```python
from build123d import *

# Parameters (mm, degrees)
F0_W     = 34.3586169891
F0_H     = 15
F1_DEPTH = 11.5
F2_DEPTH = 2.5
F3_DEPTH = 15
F5_DEPTH = 70
F6_R     = 1.75
F7_DEPTH = 50.001


with BuildPart() as f1:
    # F0 (on Top) → F1 (new body)
    with BuildSketch(Plane.XY):
        Rectangle(F0_W, F0_H)
    extrude(amount=F1_DEPTH)

    # F0 (on Top) → F2 (join)
    with BuildSketch(Plane.XY):
        Polygon((-43.5629601348, 31.9480635281), (-60, 31.9480635281), (-60, -31.9480635281), (-43.5629601348, -31.9480635281), (-17.1793084945, -13.474031764), (-17.1793084945, -10), (17.1793084945, -10), (17.1793084945, -13.474031764), (43.5629601348, -31.9480635281), (60, -31.9480635281), (60, 31.9480635281), (43.5629601348, 31.9480635281), (17.1793084945, 13.474031764), (17.1793084945, 10), (-17.1793084945, 10), (-17.1793084945, 13.474031764), align=None)
        Rectangle(F0_W, F0_H, mode=Mode.SUBTRACT)
    extrude(amount=F2_DEPTH)

    # F0 (on Top) → F3 (join)
    with BuildSketch(Plane.XY):
        Polygon((-43.5629601348, -31.9480635281), (-60, -31.9480635281), (-60, -35), (-43.5629601348, -35), (-15, -15), (15, -15), (43.5629601348, -35), (60, -35), (60, -31.9480635281), (43.5629601348, -31.9480635281), (17.1793084945, -13.474031764), (17.1793084945, -10), (-17.1793084945, -10), (-17.1793084945, -13.474031764), align=None)
        Polygon((15, 15), (-15, 15), (-43.5629601348, 35), (-60, 35), (-60, 31.9480635281), (-43.5629601348, 31.9480635281), (-17.1793084945, 13.474031764), (-17.1793084945, 10), (17.1793084945, 10), (17.1793084945, 13.474031764), (43.5629601348, 31.9480635281), (60, 31.9480635281), (60, 35), (43.5629601348, 35), align=None)
    extrude(amount=F3_DEPTH)

    # F4 (on face) → F5 (cut, through all)
    with BuildSketch(Plane.XZ.offset(35)):
        Polygon((-60, 15), (-60, 5), (-43.5629601348, 8.8385741302), (-43.5629601348, 15), align=None)
        Polygon((-43.5629601348, 15), (-43.5629601348, 8.8385741302), (-17.1793084945, 15), align=None)
        Polygon((17.1793084945, 15), (60, 5), (60, 15), align=None)
    extrude(amount=-F5_DEPTH, mode=Mode.SUBTRACT)

    # F6 (on face) → F7 (cut, through all)
    with BuildSketch(Plane.XZ.offset(15)):
        with Locations((-9.6793084945, 8.5)):
            Circle(F6_R)
        with Locations((9.6793084945, 8.5)):
            Circle(F6_R)
    extrude(amount=-F7_DEPTH, mode=Mode.SUBTRACT)


solid = f1.part
```
The listing builds one solid part. Answer for the finished solid, in the listing's coordinates (mm). A direction names the side the tool comes from. Give positions to 0.01 mm unless a question says otherwise; leave off trailing zeros. Order: outer loops, then holes, each group sorted by start corner. A loop starts at its lowest first (then second) coordinate and runs counter-clockwise, first axis right, second up. Notation, with made-up numbers: (4, 4) - (63, 4) arc R35 cw to (63, 40) - close; hole circle Ø7 at (-37, -37.5). An arc over 180 degrees is marked (long way). Answer in a Markdown table with one row per item. Add a question column.
Q1. Which of the six approach directions +Z, -Z, +X, -X, +Y, -Y give full straight-line access (tool end or side, diameter ignored) to faces 4 (the flat face through (0, -7.5, 7)), 5 (the flat face through (50, -31.948, 5)), 6 (the flat face through (-17.179, -12, 9))?
Q2. For a pull along Y with two mould halves and no side action, classify faces 1 (the flat face through (-52, -35, 3)), 2 (the flat face through (60, 0, 1)), 3 (the flat face through (-30.186, -22.582, 7.274)) as released by +Y, released by -Y, zero draft, split by the parting line, or undercut.
Q3. The part is cut by section D-D (x = -10). Determine the outline of the cut face in (y, z), then the cut area to 3 significant figures.
Q4. Find the intervals of material crossed by line 1 along Y through (x, z) = (-12, 7.25); line 2 along Y through (x, z) = (6.5, 11.75); line 3 along Z through (x, y) = (32, 1), in increasing order. Write a range as [from, to].
Q5. The part is cut by section A-A (y = 2). Determine the outline of the cut face in (x, z).
Q6. Given P1, Ø5, axis at y = 27.5, z = 7, coming from the -X side; P2, Ø12, axis at x = 45.5, y = 17.5, coming from the +Z side; P3, Ø2, axis at x = -9.68, z = 8.5, coming from the -Y side; P4, Ø1.5, axis at y = 22, z = 8, coming from the -X side, each flat-ended and moving along its own axis, determine where each tip first touches the part or whether it passes through.
Q7. The part is cut by section B-B (z = 12.75). Determine the outline of the cut face in (x, y).
Q8. The part is cut by section C-C (y = -21.5). Determine the outline of the cut face in (x, z), then the cut area to 3 significant figures.
Determined:
| question | item | result |
|---|---|---|
| 1 | face 4 | +Z, +X, -X |
| 1 | face 5 | +Z, +X |
| 1 | face 6 | +Z, -X |
| 2 | face 1 | released by -Y |
| 2 | face 2 | zero draft |
| 2 | face 3 | undercut |
| 3 | outline | (-15, 0) - (15, 0) - (15, 6.78) - (10, 6.78) - (10, 2.5) - (7.5, 2.5) - (7.5, 6.78) - (-7.5, 6.78) - (-7.5, 2.5) - (-10, 2.5) - (-10, 6.78) - (-15, 6.78) - close; (-15, 10.22) - (-10, 10.22) - (-10, 15) - (-15, 15) - close; (-7.5, 10.22) - (7.5, 10.22) - (7.5, 11.5) - (-7.5, 11.5) - close; (10, 10.22) - (15, 10.22) - (15, 15) - (10, 15) - close |
| 3 | area | 249 mm² |
| 4 | line 1 | y = [-15, -10], [-7.5, 7.5], [10, 15] |
| 4 | line 2 | y = [-15, -10], [10, 15] |
| 4 | line 3 | z = [0, 2.5] |
| 5 | outline | (-60, 0) - (60, 0) - (60, 2.5) - (17.18, 2.5) - (17.18, 11.5) - (-17.18, 11.5) - (-17.18, 2.5) - (-60, 2.5) - close; hole circle Ø3.5 at (-9.68, 8.5); hole circle Ø3.5 at (9.68, 8.5) |
| 6 | P1 | stops at x = -40.78 |
| 6 | P2 | stops at z = 2.5 |
| 6 | P3 | passes through |
| 6 | P4 | stops at x = -30.43 |
| 7 | outline | (-26.81, -23.27) - (-15, -15) - (15, -15) - (26.81, -23.27) - (26.81, -20.22) - (17.18, -13.47) - (17.18, -10) - (-17.18, -10) - (-17.18, -13.47) - (-26.81, -20.22) - close; (-26.81, 20.22) - (-17.18, 13.47) - (-17.18, 10) - (17.18, 10) - (17.18, 13.47) - (26.81, 20.22) - (26.81, 23.27) - (15, 15) - (-15, 15) - (-26.81, 23.27) - close |
| 8 | outline | (-60, 0) - (-24.28, 0) - (-24.28, 13.34) - (-28.64, 12.32) - (-28.64, 2.5) - (-60, 2.5) - close; (24.28, 0) - (60, 0) - (60, 2.5) - (28.64, 2.5) - (28.64, 12.32) - (24.28, 13.34) - close |
| 8 | area | 269 mm² |
